Geometry check sheet. Reference: the model listing, model coordinates, mm. Face numbers are marked on the shaded views. A direction names the side the tool comes from. Give positions to 0.01 mm unless a question says otherwise; leave off trailing zeros. Loops run counter-clockwise (first coordinate to the right, second up) from the corner with the lowest first, then second, coordinate; pieces in that order, holes last. Notation, with made-up numbers: (-11.5, 31.25) - (43.5, 31.25) arc R14 cw to (43.5, 56.25) - close; hole circle Ø4 at (60.5, 66). An arc over 180 degrees is marked (long way). Use a Markdown table: item, result. Add a question column.
1. Material ranges on L1, parallel to Y at x = -63, z = 0; L2, parallel to Y at x = -71.05, z = 0; L3, parallel to Y at x = 47, z = 4.5, recorded low to high.
2. Cross-section at C-C on x = 16. Enter the section's corners in (y, z), and give its area (3 significant figures).
3. Depth check by flat-ended pin: P1, Ø8, axis at x = -41, y = 9, coming from the +Z side; P2, Ø3, axis at x = -39, y = 15, coming from the +Z side; P3, Ø16.5, axis at y = -13, z = 3.5, coming from the -X side. Enter the tip coordinate at first touch or a pass-through.
4. Draft check along Z on the marked faces 3, 4, 5 and 6. Enter one of: pulls with the +Z half, pulls with the -Z half, needs draft (parallel to the pull), parting line crosses it, or undercut.
5. Cross-section at B-B on x = 58.5. Enter the section's corners in (y, z).
6. Set-up check for the marked faces 1 and 2: record each of +Z, -Z, +X, -X, +Y, -Y from which the full face is reachable in a straight line by a thin tool's end or side.
from build123d import *

# Parameters (mm, degrees)
PATTERN_CIRCULAR_1_COUNT = 6
CHAMFER_2_SIZE           = 1
CHAMFER_1_SIZE           = 2
SKETCH_5_W               = 130
SKETCH_5_H               = 10
SKETCH_6_R               = 27.5
SKETCH_6_R_2             = 23.5
CUT_EXTRUDE_1_DEPTH      = 5
CHAMFER_3_SIZE           = 1


with BuildPart() as part:
    # Эскиз1 → Повернуть1 (revolve)
    with BuildSketch(Plane.XY, mode=Mode.PRIVATE) as revolve_1_sk:
        Polygon((-75, 23.5), (-75, 47.5), (75, 47.5), (75, 23.5), (53, 23.5), (53, 21), (-53, 21), (-53, 23.5), align=None)
    revolve(revolve_1_sk.sketch.rotate(Axis((0, 0, 0), (1, 0, 0)), 90), axis=Axis((0, 0, 0), (1, 0, 0)))

    # Эскиз3 → Отверстие обработанное метчиком M61 (revolve, cut)
    with BuildSketch(Plane(origin=(-75, 37.5, 0), x_dir=(0, 0, 1), z_dir=(0, 1, 0))):
        Polygon((0, 0), (0, 17), (2.5, 15.497848452), (2.5, 0), align=None)
    hole_wizard_m61 = revolve(axis=Axis((-81.35, 37.5, 0), (1, 0, 0)), mode=Mode.SUBTRACT)

    # Круговой массив1: Отверстие обработанное метчиком M61 ×6 about axis
    pattern_circular_1_axis = Axis((0, 0, 0), (1, 0, 0))
    for i in range(1, PATTERN_CIRCULAR_1_COUNT):
        add(hole_wizard_m61.rotate(pattern_circular_1_axis, i * 360 / PATTERN_CIRCULAR_1_COUNT), mode=Mode.SUBTRACT)

    # Фаска2
    chamfer_2_edges = [part.edges().sort_by_distance(p)[0] for p in [
        (-75, 37.5, -2.5),
        (-75, 16.584936491, -33.725952642),
        (-75, -20.915063509, -31.225952642),
        (-75, -37.5, 2.5),
        (-75, -16.584936491, 33.725952642),
        (-75, 20.915063509, 31.225952642),
    ]]
    chamfer(chamfer_2_edges, length=CHAMFER_2_SIZE)

    # Фаска1
    chamfer_1_edges = [part.edges().sort_by_distance(p)[0] for p in [
        (75, 0, -23.5),
    ]]
    chamfer(chamfer_1_edges, length=CHAMFER_1_SIZE)

    # Эскиз5 → Вырез-Повернуть1 (revolve, cut)
    with BuildSketch(Plane.XY, mode=Mode.PRIVATE) as cut_revolve_1_sk:
        with Locations((10, 42.5)):
            Rectangle(SKETCH_5_W, SKETCH_5_H)
    revolve(cut_revolve_1_sk.sketch.rotate(Axis((-75, 0, 0), (1, 0, 0)), 90), axis=Axis((-75, 0, 0), (1, 0, 0)), mode=Mode.SUBTRACT)

    # Эскиз6 → Вырез-Вытянуть1 (cut)
    with BuildSketch(Plane.ZY.offset(75)):
        Circle(SKETCH_6_R)
        Circle(SKETCH_6_R_2, mode=Mode.SUBTRACT)
    extrude(amount=-CUT_EXTRUDE_1_DEPTH, mode=Mode.SUBTRACT)

    # Фаска3
    chamfer_3_edges = [part.edges().sort_by_distance(p)[0] for p in [
        (-70, 0, -23.5),
        (-75, 0, -27.5),
    ]]
    chamfer(chamfer_3_edges, length=CHAMFER_3_SIZE)


solid = part.part
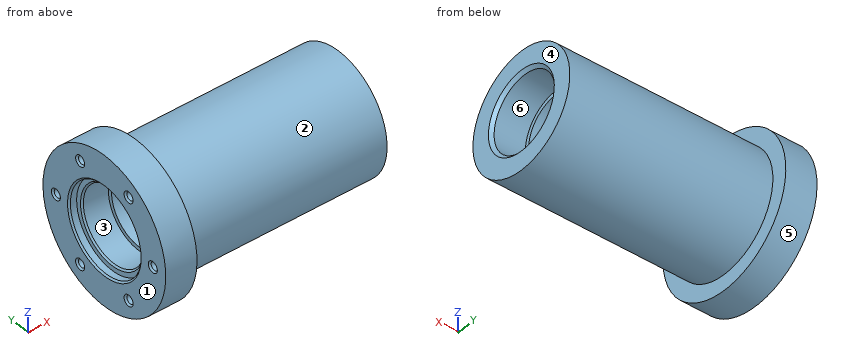
Values found:
| question | item | result |
|---|---|---|
| 1 | L1 | y = -47.5 to -40, -35 to -23.5, 23.5 to 35, 40 to 47.5 |
| 1 | L2 | y = -47.5 to -40, -35 to -27.5, 27.5 to 35, 40 to 47.5 |
| 1 | L3 | y = -37.23 to -20.51, 20.51 to 37.23 |
| 2 | outline | circle Ø75 at (0, 0); hole circle Ø42 at (0, 0) |
| 2 | area | 3,030 mm2 |
| 3 | P1 | stops at z = 37.17 |
| 3 | P2 | stops at z = 34.99 |
| 3 | P3 | stops at x = -53 |
| 4 | face 3 | undercut |
| 4 | face 4 | needs draft |
| 4 | face 5 | parting line crosses it |
| 4 | face 6 | undercut |
| 5 | outline | circle Ø75 at (0, 0); hole circle Ø47 at (0, 0) |
| 6 | face 1 | +Z, -Z, -X, +Y, -Y |
| 6 | face 2 | +X |
